Geometry: final body of the model. Coordinates: model frame, mm. Round coordinates to 2 decimals unless told otherwise and drop trailing zeros. Write each loop counter-clockwise with the first axis right and the second up, starting at its lowest first coordinate (ties: lowest second). Pieces come first, ordered by that corner, then holes.
from build123d import *

# Parameters (mm, degrees)
F0_R        = 12.4431552
F0_R_2      = 9.1690063
F1_DEPTH    = 12.7
F0_R_3      = 6.35
F2_DEPTH    = 20.32
F3_S5_R     = 9.1690063
F3_T6_DEPTH = 24


# Not quite as in the source:
# - a fillet or chamfer that OpenCascade refuses, or shapes differently, is made with other operations: its cross-section is extruded or revolved along the edge and cut away or added


with BuildPart() as f1:
    # F0 (on Right) → F1 (new body, symmetric)
    with BuildSketch(Plane.YZ):
        Circle(F0_R)
        Circle(F0_R_2, mode=Mode.SUBTRACT)
    extrude(amount=F1_DEPTH, both=True)

    # F0 (on Right) → F2 (join)
    with BuildSketch(Plane.YZ):
        Circle(F0_R_2)
        Circle(F0_R_3, mode=Mode.SUBTRACT)
    extrude(amount=F2_DEPTH)

    # F3: chamfer of 5.08 x 28.8101116437 on 1 edges, made by hand


with BuildPart() as f3_tool2:
    # F3_s3 → F3_t4 (revolve)
    with BuildSketch(Plane.XY):
        Polygon((-16.1101116437, 12.4431552), (12.7, 7.3631552), (12.7, 12.4431552), align=None)
    revolve(axis=Axis((12.7, 0, 0), (1, 0, 0)))

    # F3_s5 → F3_t6 (cut, symmetric)
    with BuildSketch(Plane.YZ.offset(-1.7)):
        Circle(F3_S5_R)
    extrude(amount=F3_T6_DEPTH, both=True, mode=Mode.SUBTRACT)


with BuildPart() as f1_1:
    add(f1.part)

    # F3_t1: cut F3_tool2
    add(f3_tool2.part, mode=Mode.SUBTRACT)

    # F4: fillet of radius 5.08 on 1 edges, made by hand

    # F4_s1 → F4_t2 (revolve, cut)
    with BuildSketch(Plane.XY):
        with BuildLine():
            ThreePointArc((15.7709003651, 9.1690063), (18.44676957, 8.4071220926), (20.32, 6.35))
            Line((20.32, 6.35), (20.32, 9.1690063))
            Line((20.32, 9.1690063), (15.7709003651, 9.1690063))
        make_face()
    revolve(axis=Axis((20.32, 0, 0), (1, 0, 0)), mode=Mode.SUBTRACT)


solid = f1_1.part
1) Section A-A on x = 11. Output: boundary loops of the cut face in (y, z), plus the area to 3 significant figures.
2) First-contact query: P1, Ø4, axis at x = -5, y = 5.5, coming from the -Z side; P2, Ø4, axis at x = -6, z = 9.5, coming from the +Y side; P3, Ø4, axis at x = 10, y = -7.5, coming from the +Z side. Flat tips, straight axial feed; report the tip coordinate or a pass-through.
3) Line query: probe 1 along Z at (x, y) = (15.25, 0); probe 2 along Y at (x, z) = (9, 4.75); probe 3 along Z at (x, y) = (12, 5.5). Output: solid intervals per line, ascending.
4) Section B-B on x = -2. Output: boundary loops of the cut face in (y, z), plus the area to 3 significant figures.
5) Draft query along Y for faces 1 (the flat face through (-12.7, 3, -9)), 2 (the conical face through (-3.33, 9.413, -3.903)), 3 (the cylindrical face through (10.02, -1.38, -6.2)). Return one class per face: pulls with the +Y half, pulls with the -Y half, needs draft (parallel to the pull), parting line crosses it, or undercut.
Filled in:
1. outline: circle Ø18.34 at (0, 0); hole circle Ø12.7 at (0, 0)
1. area: 137 mm2
2. P1: stops at z = -9.97
2. P2: stops at y = 7.64
2. P3: stops at z = 7.34
3. probe 1: z = -9.17 to -6.35, 6.35 to 9.17
3. probe 2: y = -7.84 to -4.21, 4.21 to 7.84
3. probe 3: z = -7.34 to -3.17, 3.17 to 7.34
4. outline: circle Ø19.91 at (0, 0); hole circle Ø18.34 at (0, 0)
4. area: 47.2 mm2
5. face 1: needs draft
5. face 2: parting line crosses it
5. face 3: undercut
